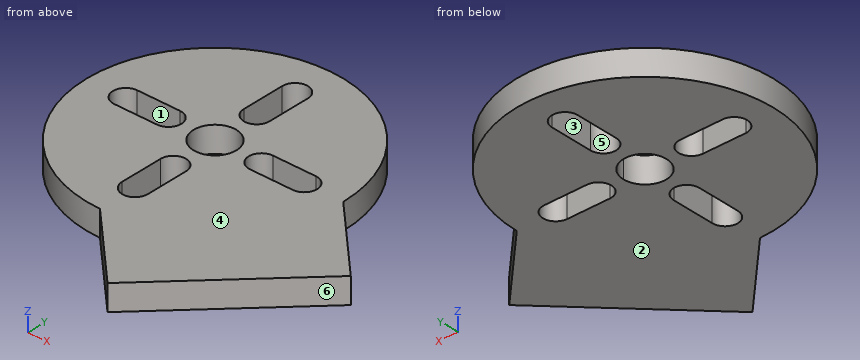
```python
from build123d import *

# Parameters (mm, degrees)
F1_DEPTH = 3


with BuildPart() as f1:
    # F0 (on Top) → F1 (new body)
    with BuildSketch(Plane.XY):
        with BuildLine():
            Line((-47.178107, 62.178107), (-55.710678, 70.710678))
            ThreePointArc((-55.710678, 70.710678), (-81.31728, 81.31728), (-70.710678, 55.710678))
            Line((-70.710678, 55.710678), (-62.178107, 47.178107))
            Line((-62.178107, 47.178107), (-47.178107, 62.178107))
        make_face()
        with BuildLine():
            ThreePointArc((-72.210678, 65.270315), (-70.710678, 66.770315), (-69.210678, 65.270315))
            Line((-69.210678, 65.270315), (-69.210678, 60.270315))
            ThreePointArc((-69.210678, 60.270315), (-70.710678, 58.770315), (-72.210678, 60.270315))
            Line((-72.210678, 60.270315), (-72.210678, 65.270315))
        make_face(mode=Mode.SUBTRACT)
        with BuildLine():
            ThreePointArc((-76.151041, 72.210678), (-74.651041, 70.710678), (-76.151041, 69.210678))
            Line((-76.151041, 69.210678), (-81.151041, 69.210678))
            ThreePointArc((-81.151041, 69.210678), (-82.651041, 70.710678), (-81.151041, 72.210678))
            Line((-81.151041, 72.210678), (-76.151041, 72.210678))
        make_face(mode=Mode.SUBTRACT)
        with BuildLine():
            ThreePointArc((-68.942911, 72.478445), (-68.400979, 71.667387), (-68.210678, 70.710678))
            ThreePointArc((-68.210678, 70.710678), (-69.75397, 68.400979), (-72.478445, 68.942911))
            ThreePointArc((-72.478445, 68.942911), (-72.478445, 72.478445), (-68.942911, 72.478445))
        make_face(mode=Mode.SUBTRACT)
        with BuildLine():
            Line((-69.210678, 81.151041), (-69.210678, 76.151041))
            ThreePointArc((-69.210678, 76.151041), (-70.710678, 74.651041), (-72.210678, 76.151041))
            Line((-72.210678, 76.151041), (-72.210678, 81.151041))
            ThreePointArc((-72.210678, 81.151041), (-70.710678, 82.651041), (-69.210678, 81.151041))
        make_face(mode=Mode.SUBTRACT)
        with BuildLine():
            Line((-60.270315, 69.210678), (-65.270315, 69.210678))
            ThreePointArc((-65.270315, 69.210678), (-66.770315, 70.710678), (-65.270315, 72.210678))
            Line((-65.270315, 72.210678), (-60.270315, 72.210678))
            ThreePointArc((-60.270315, 72.210678), (-58.770315, 70.710678), (-60.270315, 69.210678))
        make_face(mode=Mode.SUBTRACT)
    extrude(amount=F1_DEPTH)


solid = f1.part
```
The model under review builds one solid part; all positions refer to its coordinate system, in mm. Face numbers are marked on the shaded views. A direction names the side the tool comes from. Give positions to 0.01 mm unless a question says otherwise; leave off trailing zeros. Write each loop counter-clockwise with the first axis right and the second up, starting at its lowest first coordinate (ties: lowest second). Pieces come first, ordered by that corner, then holes. Notation, with made-up numbers: M -19,49.5 L 4,49.5 A28 ccw 4,73.5 Z; hole C 80,9 d11. An arc over 180 degrees is marked long. Write item = value, one per line. Start each with the question number.
Q1. For line 1 (Y direction, x = -71.5, z = 1); line 2 (X direction, y = 69.5, z = 1.2); line 3 (X direction, y = 72, z = 0.1), list the stretches that pass through material, from the lowest coordinate up.
Q2. We need section C-C (x = -77.5). State the section outline as (y, z) points.
Q3. Mouldability with a two-part tool opening along X and no side actions: class the marked faces 3, 4, 5 and 6 as released by +X, released by -X, zero draft, split by the parting line, or undercut.
Q4. We need section A-A (z = 2.3). State the section outline as (x, y) points, plus the area to 3 significant figures.
Q5. Clearance check with flat-ended pins moving along their axes: pin 1 (0.9 mm diameter, centred on x = -63, z = 2, fed in from +Y); pin 2 (0.9 mm diameter, centred on y = 61.5, z = 1.5, fed in from -X); pin 3 (0.9 mm diameter, centred on x = -79, z = 2, fed in from +Y). State where each tip first meets the part, or that it passes through.
Q6. We need section D-D (x = -53). State the section outline as (y, z) points, plus the area to 3 significant figures.
Q7. Machinability: for the marked faces 1 and 2, which of the approach directions +Z, -Z, +X, -X, +Y, -Y give a long, thin tool a straight path to every point of the face, cutting with its end or side? Answer none if there is none.
Q8. We need section B-B (y = 75.5). State the section outline as (x, z) points.
Result set:
q1.line_1 = 55.73 to 58.99, 66.55 to 68.34, 73.08 to 74.88, 82.43 to 85.69
q1.line_2 = -85.66 to -82.04, -75.27 to -72.9, -68.52 to -66.16, -59.38 to -54.5
q1.line_3 = -85.66 to -81.92, -75.38 to -72.85, -68.57 to -66.04, -59.5 to -55.77
q2.outline = M 57.34,0 L 69.21,0 L 69.21,3 L 57.34,3 Z; M 72.21,0 L 84.09,0 L 84.09,3 L 72.21,3 Z
q3.face_3 = undercut
q3.face_4 = zero draft
q3.face_5 = undercut
q3.face_6 = released by +X
q4.outline = M -70.71,55.71 L -62.18,47.18 L -47.18,62.18 L -55.71,70.71 A15 ccw long Z; hole M -81.15,69.21 L -76.15,69.21 A1.5 ccw -76.15,72.21 L -81.15,72.21 A1.5 ccw Z; hole M -72.21,60.27 A1.5 ccw -69.21,60.27 L -69.21,65.27 A1.5 ccw -72.21,65.27 Z; hole M -72.21,76.15 A1.5 ccw -69.21,76.15 L -69.21,81.15 A1.5 ccw -72.21,81.15 Z; hole M -68.94,72.48 A2.5 ccw long -68.21,70.71 A2.5 ccw Z; hole M -65.27,69.21 L -60.27,69.21 A1.5 ccw -60.27,72.21 L -65.27,72.21 A1.5 ccw Z
q4.area = 791 mm2
q5.pin_1 = 83.84
q5.pin_2 = -82.89
q5.pin_3 = 83.5
q6.outline = M 56.36,0 L 68,0 L 68,3 L 56.36,3 Z
q6.area = 34.9 mm2
q7.face_1 = +Z, -Z
q7.face_2 = -Z, +X, -X, +Y, -Y
q8.outline = M -84.93,0 L -72.06,0 L -72.06,3 L -84.93,3 Z; M -69.36,0 L -56.5,0 L -56.5,3 L -69.36,3 Z
